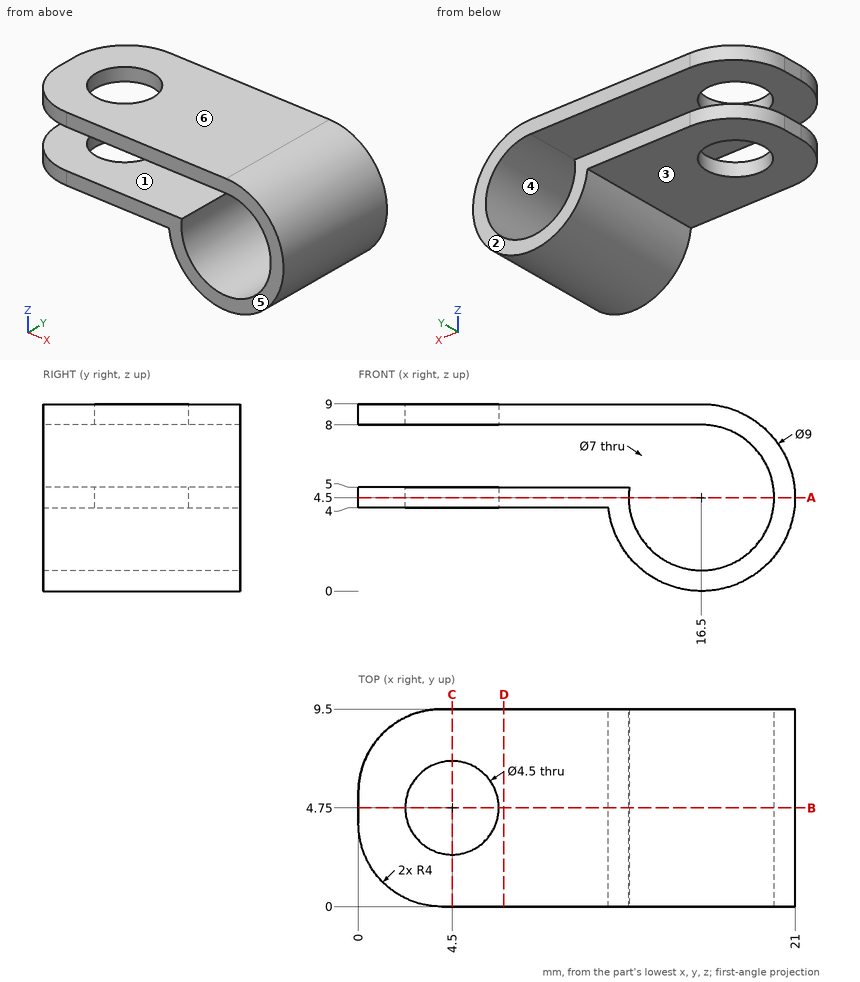
Here's the drawing with two shaded views (mm, measured from the low corner). I have some questions. A direction names the side the tool comes from. Coordinates: 2 decimals unless noted, no trailing zeros. Loops run counter-clockwise (first coordinate to the right, second up) from the corner with the lowest first, then second, coordinate; pieces in that order, holes last. Notation, with made-up numbers: (59, -7.5) -> (118, -7.5) arc R12 ccw to (118, 7.5) -> close; hole circle Ø3 at (22, 41). An arc over 180 degrees is marked (long way). Answer in a Markdown table with one row per item.
(1) If I drill on probe 1 along Z at (x, y) = (9.75, 4.5); probe 2 along Y at (x, z) = (4.5, 4.7); probe 3 along Z at (x, y) = (16.5, 4.5), over which ranges is the centre line in solid material (lowest first)?
Results found:
| item | result |
|---|---|
| probe 1 | z = 4 to 5, 8 to 9 |
| probe 2 | y = 0 to 2.5, 7 to 9.5 |
| probe 3 | z = 0 to 1, 8 to 9 |
(2) Imagine slicing it at D-D (x = 7). List the corners of the cut face in (y, z) for me.
Results found:
| item | result |
|---|---|
| outline | (0, 4) -> (9.5, 4) -> (9.5, 5) -> (0, 5) -> close; (0, 8) -> (9.5, 8) -> (9.5, 9) -> (0, 9) -> close |
(3) Thinking about a two-plate mould opening in Z: for the marked faces 4, 5 and 6, which applies, released by +Z, released by -Z, zero draft, split by the parting line, or undercut?
Results found:
| item | result |
|---|---|
| face 4 | undercut |
| face 5 | zero draft |
| face 6 | released by +Z |
(4) Imagine slicing it at A-A (z = 4.5). List the corners of the cut face in (x, y) for me.
Results found:
| item | result |
|---|---|
| outline | (0, 4) arc R4 ccw to (4, 0) -> (13, 0) -> (13, 9.5) -> (4, 9.5) arc R4 ccw to (0, 5.5) -> close; (20, 0) -> (21, 0) -> (21, 9.5) -> (20, 9.5) -> close; hole circle Ø4.5 at (4.5, 4.75) |
(5) Imagine slicing it at B-B (y = 4.75). List the corners of the cut face in (x, z) for me.
Results found:
| item | result |
|---|---|
| outline | (0, 4) -> (2.25, 4) -> (2.25, 5) -> (0, 5) -> close; (0, 8) -> (2.25, 8) -> (2.25, 9) -> (0, 9) -> close; (6.75, 4) -> (12.03, 4) arc R4.5 ccw (long way) to (16.5, 9) -> (6.75, 9) -> (6.75, 8) -> (16.5, 8) arc R3.5 cw (long way) to (13.04, 5) -> (6.75, 5) -> close |
(6) For the marked faces 1, 2 and 3, which set-ups out of +Z, -Z, +X, -X, +Y, -Y let a thin tool reach every point of the face, with its end or its side?
Results found:
| item | result |
|---|---|
| face 1 | -X, +Y, -Y |
| face 2 | +Z, -Z, +X, -X, +Y |
| face 3 | -Z, -X, +Y, -Y |
(7) Imagine slicing it at C-C (x = 4.5). List the corners of the cut face in (y, z) for me, plus the area to 3 significant figures.
Results found:
| item | result |
|---|---|
| outline | (0, 4) -> (2.5, 4) -> (2.5, 5) -> (0, 5) -> close; (0, 8) -> (2.5, 8) -> (2.5, 9) -> (0, 9) -> close; (7, 4) -> (9.5, 4) -> (9.5, 5) -> (7, 5) -> close; (7, 8) -> (9.5, 8) -> (9.5, 9) -> (7, 9) -> close |
| area | 10.0 mm^2 |
(8) Will these pins go through, and if not, where does the flat tip stop? pin 1 Ø5 at (x, y) = (8.5, 4.5) entering from -Z; pin 2 Ø4 at (x, y) = (4.5, 4.75) entering from +Z; pin 3 Ø2 at (y, z) = (2, 6) entering from +X.
Results found:
| item | result |
|---|---|
| pin 1 | stops at z = 4 |
| pin 2 | passes through |
| pin 3 | stops at x = 20.97 |
